from build123d import *

# Parameters (mm, degrees)
F1_DEPTH = 25.4
F2_T     = -3.175
F3_R     = 6.35
F5_W     = 12.7
F5_H     = 6.35
F6_DEPTH = 21.844


# Not quite as in the source:
# - a feature names something its author has since deleted; it is built from what else it names


with BuildPart() as f1:
    # F0 (on Top) → F1 (new body)
    with BuildSketch(Plane.XY):
        with BuildLine():
            Line((58.0965084505, 62.5356453779), (-58.0965084505, 62.5356453779))
            ThreePointArc((-58.0965084505, 62.5356453779), (-66.1787389595, 59.1878758868), (-69.5265084505, 51.1056453779))
            Line((-69.5265084505, 51.1056453779), (-69.5265084505, -27.1992570698))
            ThreePointArc((-69.5265084505, -27.1992570698), (-67.0115325937, -35.1957139026), (-60.3721316603, -40.3130159932))
            ThreePointArc((-60.3721316603, -40.3130159932), (0, -51.0474727306), (60.3721316603, -40.3130159932))
            ThreePointArc((60.3721316603, -40.3130159932), (67.0115325937, -35.1957139026), (69.5265084505, -27.1992570698))
            Line((69.5265084505, -27.1992570698), (69.5265084505, 51.1056453779))
            ThreePointArc((69.5265084505, 51.1056453779), (66.1787389595, 59.1878758868), (58.0965084505, 62.5356453779))
        make_face()
    extrude(amount=F1_DEPTH)

    # F2
    f2_openings = [f1.faces().sort_by_distance(p)[0] for p in [
        (0, 7.919531, 25.4),
    ]]
    offset(amount=F2_T, openings=f2_openings)

    # F3
    f3_edges = [f1.edges().sort_by_distance(p)[0] for p in [
        (69.526508, 11.953194, 0),
        (66.178739, 59.187876, 0),
        (0, 62.535645, 0),
        (-66.178739, 59.187876, 0),
        (-69.526508, 11.953194, 0),
        (-67.011533, -35.195714, 0),
        (0, -51.047473, 0),
        (67.011533, -35.195714, 0),
    ]]
    fillet(f3_edges, radius=F3_R)

    # F5 (on offset) → F6 (join)
    with BuildSketch(Plane.XY.offset(25.4)):
        with Locations((-53.0805146158, 57.0815077901)):
            Rectangle(F5_W, F5_H)
        with Locations((53.0805146158, 57.0815077901)):
            Rectangle(F5_W, F5_H)
        Polygon((-41.1578565836, -33.773638308), (-58.6946308613, -33.773638308), (-60.6418885291, -37.9110425711), (-53.9016760886, -40.266495198), (-41.1578565836, -43.8219420612), align=None)
        Polygon((60.6418885291, -37.9110425711), (58.6946308613, -33.773638308), (41.1578565836, -33.773638308), (41.1578565836, -43.8219420612), (53.9016760886, -40.266495198), align=None)
    extrude(amount=-F6_DEPTH)


solid = f1.part
Here's how the part is built. I have some questions about the finished solid (model axes, mm). A direction names the side the tool comes from. Coordinates: 2 decimals unless noted, no trailing zeros. Loops run counter-clockwise (first coordinate to the right, second up) from the corner with the lowest first, then second, coordinate; pieces in that order, holes last.
1. For faces 1 (the flat face through (-53, 57, 3.556)), 2 (the cylindrical face through (-0.863, -51.045, 15.742)), 3 (the flat face through (-50, -33.774, 15)), which set-ups out of +Z, -Z, +X, -X, +Y, -Y let a thin tool reach every point of the face, with its end or its side?
2. If we mould it in two halves opening along Z, with no side actions, what happens to faces 4 (the flat face through (53, 57, 3.556)), 5 (the flat face through (-49, -37, 3.556)), 6 (the cylindrical face through (67.716, 12.501, 1.91)), 7 (the flat face through (66.352, 11, 14))? For each: pulls with the +Z half, pulls with the -Z half, needs draft (parallel to the pull), parting line crosses it, or undercut.
3. I need wall thicknesses on L1, parallel to Z at x = -54, y = 56.5 (3 decimals); L2, parallel to X at y = -18.5, z = 24.75; L3, parallel to Y at x = -0.5, z = 9. Which ranges of each line are inside material? Lowest first, please.
4. For P1, Ø6, axis at y = 57.5, z = 14, coming from the -X side; P2, Ø2.5, axis at x = 51.5, y = -38.5, coming from the -Z side; P3, Ø6, axis at y = 57, z = 13.5, coming from the +X side, each with a flat end and sliding along its axis, tell me the tip position at first contact or that it passes through.
5. Imagine slicing it at A-A, the plane z = 10.25. Please give me the cut outline in (x, y) (1 decimal).
Taken from the geometry:
1. face 1: none
1. face 2: +Z, -Z, -Y
1. face 3: +Z
2. face 4: undercut
2. face 5: undercut
2. face 6: pulls with the -Z half
2. face 7: needs draft
3. L1: z = 0.008 to 3.175, 3.556 to 25.4
3. L2: x = -69.53 to -66.35, 66.35 to 69.53
3. L3: y = -51.05 to -47.87, 59.36 to 62.54
4. P1: stops at x = -69.01
4. P2: stops at z = 0.02
4. P3: stops at x = 69.15
5. outline: (-69.5, -27.2) arc R14 ccw to (-60.4, -40.3) arc R175.1 ccw to (60.4, -40.3) arc R14 ccw to (69.5, -27.2) - (69.5, 51.1) arc R11.4 ccw to (58.1, 62.5) - (-58.1, 62.5) arc R11.4 ccw to (-69.5, 51.1) - close; hole (-66.4, -27.2) arc R10.8 ccw to (-60.2, -36.9) - (-58.7, -33.8) - (-41.2, -33.8) - (-41.2, -42.9) arc R172 ccw to (41.2, -42.9) - (41.2, -33.8) - (58.7, -33.8) - (60.2, -36.9) arc R10.8 ccw to (66.4, -27.2) - (66.4, 51.1) arc R8.3 ccw to (59.4, 59.3) - (59.4, 53.9) - (46.7, 53.9) - (46.7, 59.4) - (-46.7, 59.4) - (-46.7, 53.9) - (-59.4, 53.9) - (-59.4, 59.3) arc R8.3 ccw to (-66.4, 51.1) - close
